```python
from build123d import *

# Parameters (mm, degrees)
SKETCH1_W           = 159
SKETCH1_H           = 38
SKETCH1_R           = 1.5
SKETCH1_R_2         = 10.55
SKETCH1_R_3         = 6
BOSS_EXTRUDE1_DEPTH = 10
FILLET1_R           = 10


with BuildPart() as part:
    # Sketch1 → Boss-Extrude1 (new body)
    with BuildSketch(Plane(origin=(0, 0, 0), x_dir=(1, 0, 0), z_dir=(0, 1, 0))):
        Rectangle(SKETCH1_W, SKETCH1_H)
        with Locations((9, 15.5)):
            Circle(SKETCH1_R, mode=Mode.SUBTRACT)
        with Locations((-9, 15.5)):
            Circle(SKETCH1_R, mode=Mode.SUBTRACT)
        with Locations((-9, -15.5)):
            Circle(SKETCH1_R, mode=Mode.SUBTRACT)
        with Locations((9, -15.5)):
            Circle(SKETCH1_R, mode=Mode.SUBTRACT)
        with Locations((-67.5, 0)):
            Circle(SKETCH1_R_2, mode=Mode.SUBTRACT)
        with Locations((67.5, 0)):
            Circle(SKETCH1_R_2, mode=Mode.SUBTRACT)
        with Locations((42.5, 0)):
            Circle(SKETCH1_R_3, mode=Mode.SUBTRACT)
    extrude(amount=BOSS_EXTRUDE1_DEPTH)

    # Fillet1
    fillet1_edges = [part.edges().sort_by_distance(p)[0] for p in [
        (79.5, 5, 19),
        (-79.5, 5, 19),
        (-79.5, 5, -19),
        (79.5, 5, -19),
    ]]
    fillet(fillet1_edges, radius=FILLET1_R)


solid = part.part
```
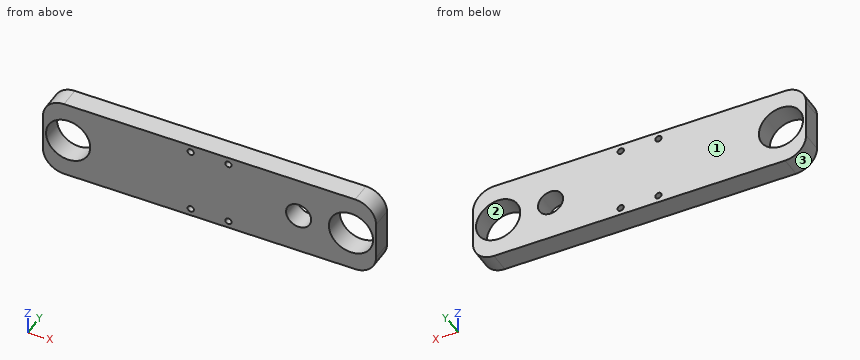
Source: CAD feature listing. Evaluate the final solid. Frame: model axes, mm. Face numbers are marked on the shaded views. Coordinates: 2 decimals unless noted, no trailing zeros. Write each loop counter-clockwise with the first axis right and the second up, starting at its lowest first coordinate (ties: lowest second). Pieces come first, ordered by that corner, then holes. Notation, with made-up numbers: (-2.5, -39.5) -> (14.5, -39.5) arc R21 ccw to (14.5, -3.5) -> close; hole circle Ø10 at (87.5, 46). An arc over 180 degrees is marked (long way). Return JSON: item names as keys, results as strings. Group by question number.
1) Ray query, line 1 along Z through (x, y) = (-9, 6); line 2 along X through (y, z) = (7, 7.5); line 3 along X through (y, z) = (4, 15.5). Return the intervals inside material, ascending.
2) Section query B-B, the plane z = 0. Return loops of the section in (x, y).
3) Contact query for flat-ended pins moving along their axis: P1, Ø2, axis at y = 1.5, z = 11, coming from the -X side; P2, Ø1.8, axis at x = -9, z = 15.5, coming from the +Y side (3 decimals). Output: stop coordinate, or through.
4) Section query A-A, the plane x = 42.5. Return loops of the section in (y, z).
5) Section query D-D, the plane x = -9. Return loops of the section in (y, z), plus the area to 3 significant figures.
6) Section query C-C, the plane y = 3.5. Return loops of the section in (x, z).
7) Mould query, pull axis X, two halves, no side actions, for the marked faces 1, 2 and 3. Classes: +X half, -X half, draft (parallel to the pull), parting line (faces both ways), or undercut.
From the geometry:
{
 "1": {"line 1": "-19 to -17, -14 to 14, 17 to 19", "line 2": "-79.5 to -74.92, -60.08 to 60.08, 74.92 to 79.5", "line 3": "-77.1 to -10.5, -7.5 to 7.5, 10.5 to 77.1"},
 "2": {"outline": "(-79.5, 0) -> (-78.05, 0) -> (-78.05, 10) -> (-79.5, 10) -> close; (-56.95, 0) -> (36.5, 0) -> (36.5, 10) -> (-56.95, 10) -> close; (48.5, 0) -> (56.95, 0) -> (56.95, 10) -> (48.5, 10) -> close; (78.05, 0) -> (79.5, 0) -> (79.5, 10) -> (78.05, 10) -> close"},
 "3": {"P1": "x = -79.45", "P2": "through"},
 "4": {"outline": "(0, -19) -> (10, -19) -> (10, -6) -> (0, -6) -> close; (0, 6) -> (10, 6) -> (10, 19) -> (0, 19) -> close"},
 "5": {"outline": "(0, -19) -> (10, -19) -> (10, -17) -> (0, -17) -> close; (0, -14) -> (10, -14) -> (10, 14) -> (0, 14) -> close; (0, 17) -> (10, 17) -> (10, 19) -> (0, 19) -> close", "area": "320 mm²"},
 "6": {"outline": "(-79.5, -9) arc R10 ccw to (-69.5, -19) -> (69.5, -19) arc R10 ccw to (79.5, -9) -> (79.5, 9) arc R10 ccw to (69.5, 19) -> (-69.5, 19) arc R10 ccw to (-79.5, 9) -> close; hole circle Ø21.1 at (-67.5, 0); hole circle Ø3 at (-9, -15.5); hole circle Ø3 at (-9, 15.5); hole circle Ø3 at (9, -15.5); hole circle Ø3 at (9, 15.5); hole circle Ø12 at (42.5, 0); hole circle Ø21.1 at (67.5, 0)"},
 "7": {"face 1": "draft", "face 2": "undercut", "face 3": "-X half"}
}
